```python
from build123d import *

# Parameters (mm, degrees)
F0_W      = 58
F0_H      = 152
F1_DEPTH  = 42
F3_DEPTH  = 25
F4_DEPTH  = 25
F5_W      = 130
F5_H      = 3
F6_DEPTH  = 58
F7_DEPTH  = 30
F8_W      = 9.5
F8_H      = 35
F9_DEPTH  = 29.4
F10_W     = 9.5
F10_H     = 23.6
F11_DEPTH = 82
F12_SIZE  = 2
F13_W     = 40
F13_H     = 92
F14_DEPTH = 26.4


with BuildPart() as f1:
    # F0 (on Top) → F1 (new body)
    with BuildSketch(Plane.XY):
        with Locations((-19.09, 37.088177)):
            Rectangle(F0_W, F0_H)
    extrude(amount=F1_DEPTH)

    # F2 (on face) → F3 (cut)
    with BuildSketch(Plane.XY.offset(42)):
        with BuildLine():
            Line((-20.84, 88.588177), (-20.84, 92.066549))
            ThreePointArc((-20.84, 92.066549), (-15.94, 98.088177), (-20.84, 104.109805))
            Line((-20.84, 104.109805), (-20.84, 107.588177))
            Line((-20.84, 107.588177), (-23.34, 107.588177))
            Line((-23.34, 107.588177), (-23.34, 104.109805))
            ThreePointArc((-23.34, 104.109805), (-28.24, 98.088177), (-23.34, 92.066549))
            Line((-23.34, 92.066549), (-23.34, 88.588177))
            Line((-23.34, 88.588177), (-20.84, 88.588177))
        make_face()
    extrude(amount=-F3_DEPTH, mode=Mode.SUBTRACT)

    # F2 (on face) → F4 (cut)
    with BuildSketch(Plane.XY.offset(42)):
        with BuildLine():
            Line((-20.84, -31.061823), (-20.84, -29.933451))
            ThreePointArc((-20.84, -29.933451), (-17.741293, -28.26053), (-16.068372, -25.161823))
            Line((-16.068372, -25.161823), (-14.94, -25.161823))
            Line((-14.94, -25.161823), (-14.94, -22.661823))
            Line((-14.94, -22.661823), (-16.068372, -22.661823))
            ThreePointArc((-16.068372, -22.661823), (-17.741293, -19.563116), (-20.84, -17.890195))
            Line((-20.84, -17.890195), (-20.84, -16.761823))
            Line((-20.84, -16.761823), (-23.34, -16.761823))
            Line((-23.34, -16.761823), (-23.34, -17.890195))
            ThreePointArc((-23.34, -17.890195), (-26.438706, -19.563116), (-28.111627, -22.661823))
            Line((-28.111627, -22.661823), (-29.24, -22.661823))
            Line((-29.24, -22.661823), (-29.24, -25.161823))
            Line((-29.24, -25.161823), (-28.111627, -25.161823))
            ThreePointArc((-28.111627, -25.161823), (-26.438706, -28.26053), (-23.34, -29.933451))
            Line((-23.34, -29.933451), (-23.34, -31.061823))
            Line((-23.34, -31.061823), (-20.84, -31.061823))
        make_face()
    extrude(amount=-F4_DEPTH, mode=Mode.SUBTRACT)

    # F5 (on face) → F6 (cut, through all)
    with BuildSketch(Plane.YZ.offset(9.91)):
        with Locations((37.088177, 14.1)):
            Rectangle(F5_W, F5_H)
    extrude(amount=-F6_DEPTH, mode=Mode.SUBTRACT)

    # F5 (on face) → F7 (join)
    with BuildSketch(Plane.YZ.offset(9.91)):
        Polygon((102.088177, 12.6), (-27.911823, 12.6), (-38.911823, 12.6), (-38.911823, 0), (113.088177, 0), (113.088177, 12.6), align=None)
    extrude(amount=F7_DEPTH)

    # F8 (on face) → F9 (cut, through all)
    with BuildSketch(Plane.XY.offset(42)):
        with Locations((5.16, -21.411823)):
            Rectangle(F8_W, F8_H)
        with Locations((5.16, 95.588177)):
            Rectangle(F8_W, F8_H)
    extrude(amount=-F9_DEPTH, mode=Mode.SUBTRACT)

    # F10 (on face) → F11 (cut, through all)
    with BuildSketch(Plane.XZ.offset(3.911823)):
        with Locations((5.16, 27.4)):
            Rectangle(F10_W, F10_H)
    extrude(amount=-F11_DEPTH, mode=Mode.SUBTRACT)

    # F12
    f12_edges = [f1.edges().sort_by_distance(p)[0] for p in [
        (-4.09, -38.911823, 0),
        (-48.09, -38.911823, 21),
        (-23.84, -38.911823, 42),
        (0.41, -38.911823, 27.3),
        (20.16, -38.911823, 12.6),
        (39.91, -38.911823, 6.3),
        (39.91, 113.088177, 6.3),
        (20.16, 113.088177, 12.6),
        (0.41, 113.088177, 27.3),
        (-23.84, 113.088177, 42),
        (-48.09, 113.088177, 21),
        (-4.09, 113.088177, 0),
        (39.91, 37.088177, 12.6),
        (39.91, 37.088177, 0),
    ]]
    chamfer(f12_edges, length=F12_SIZE)

    # F13 (on face) → F14 (cut, through all)
    with BuildSketch(Plane.XY.offset(42)):
        with Locations((-28.09, 37.088177)):
            Rectangle(F13_W, F13_H)
    extrude(amount=-F14_DEPTH, mode=Mode.SUBTRACT)


solid = f1.part
```
The listing builds one solid part. Answer for the finished solid, in the listing's coordinates (mm). A direction names the side the tool comes from. Give positions to 0.01 mm unless a question says otherwise; leave off trailing zeros. Order: outer loops, then holes, each group sorted by start corner. A loop starts at its lowest first (then second) coordinate and runs counter-clockwise, first axis right, second up.
Item 1: The part is cut by section B-B, the plane y = 52. Give the vertices of the cut face in (x, z).
From the geometry:
outline: (-48.09, 0) - (37.91, 0) - (39.91, 2) - (39.91, 10.6) - (37.91, 12.6) - (-48.09, 12.6) - close; (-8.09, 15.6) - (0.41, 15.6) - (0.41, 39.2) - (9.91, 39.2) - (9.91, 42) - (-8.09, 42) - close
Item 2: For a pull along X with two mould halves and no side action, classify faces 5 (the face through (-7, 36, 15.6)), 6 (the face through (-15.94, 97.97, 29.68)) as pulls with the +X half, pulls with the -X half, needs draft (parallel to the pull), parting line crosses it, or undercut.
From the geometry:
face 5: needs draft
face 6: undercut
Item 3: Find the intervals of material crossed by probe 1 along Z at (x, y) = (-1, 47); probe 2 along Z at (x, y) = (6.5, 59.5); probe 3 along Y at (x, z) = (-9.5, 36), in increasing order.
From the geometry:
probe 1: z = 0 to 12.6, 15.6 to 42
probe 2: z = 0 to 12.6, 39.2 to 42
probe 3: y = -38.91 to -8.91, 83.09 to 113.09
Item 4: The part is cut by section A-A, the plane x = -5.5. Give the vertices of the cut face in (y, z), and give its area (3 significant figures).
From the geometry:
outline: (-38.91, 2) - (-36.91, 0) - (111.09, 0) - (113.09, 2) - (113.09, 40) - (111.09, 42) - (-36.91, 42) - (-38.91, 40) - close; hole (-27.91, 12.6) - (102.09, 12.6) - (102.09, 15.6) - (-27.91, 15.6) - close
area: 5,990 mm2
Item 5: Which of the six approach directions +Z, -Z, +X, -X, +Y, -Y give full straight-line access (tool end or side, diameter ignored) to faces 1 (the face through (5, -3.912, 41)), 2 (the face through (-26.5, -28.2, 29.7)), 3 (the face through (5, 78.088, 41)), 4 (the face through (-28, -8.912, 29))?
From the geometry:
face 1: +Z, +X, -Y
face 2: +Z
face 3: +Z, +X, +Y
face 4: +Z, -X
Item 6: The part is cut by section D-D, the plane x = -34.5. Give the vertices of the cut face in (y, z).
From the geometry:
outline: (-38.91, 2) - (-36.91, 0) - (111.09, 0) - (113.09, 2) - (113.09, 40) - (111.09, 42) - (83.09, 42) - (83.09, 15.6) - (102.09, 15.6) - (102.09, 12.6) - (-27.91, 12.6) - (-27.91, 15.6) - (-8.91, 15.6) - (-8.91, 42) - (-36.91, 42) - (-38.91, 40) - close
Item 7: The part is cut by section C-C, the plane x = 8. Give the vertices of the cut face in (y, z), and give its area (3 significant figures).
From the geometry:
outline: (-38.91, 2) - (-36.91, 0) - (111.09, 0) - (113.09, 2) - (113.09, 10.6) - (111.09, 12.6) - (-36.91, 12.6) - (-38.91, 10.6) - close; (-3.91, 39.2) - (78.09, 39.2) - (78.09, 42) - (-3.91, 42) - close
area: 2,140 mm2
Item 8: Given pin 1 Ø1.2 at (y, z) = (-24.5, 26.5) entering from +X; pin 2 Ø4 at (y, z) = (-3.5, 18.5) entering from -X; pin 3 Ø23.5 at (y, z) = (49.5, 30) entering from +X, each flat-ended and moving along its own axis, determine where each tip first touches the part or whether it passes through.
From the geometry:
pin 1: stops at x = 0.41
pin 2: stops at x = -8.09
pin 3: stops at x = 9.91
